For this review, take the finished solid that the model builds, in its own axes (mm). Give positions to 0.01 mm unless a question says otherwise; leave off trailing zeros. Write each loop counter-clockwise with the first axis right and the second up, starting at its lowest first coordinate (ties: lowest second). Pieces come first, ordered by that corner, then holes.
Q1. We need section C-C (z = 1.05). Write out the cut boundary in (x, y), then the cut area to 3 significant figures.
Q2. We need section A-A (y = 10). Write out the cut boundary in (x, z), then the cut area to 3 significant figures.
Q3. Insertion check: P1, Ø1.5, axis at x = -17, z = 1, coming from the -Y side; P2, Ø5, axis at x = -10, y = 10, coming from the +Z side. Each pin has a flat end and moves straight along its axis. Give the tip position at first contact, or say it passes through.
Q4. We need section B-B (x = -10). Write out the cut boundary in (y, z).
Q5. We need section D-D (y = 55). Write out the cut boundary in (x, z).
Q6. For line 1 (Y direction, x = -10, z = 0.6); line 2 (Y direction, x = -12.5, z = 0.25); line 3 (X direction, y = 13.5, z = 2.2), list the stretches that pass through material, from the lowest coordinate up.
Autodesk Inventor part; units mm, degrees
ref_plane "YZ Plane" through (0, 0, 0) normal (1, 0, 0) x (0, 1, 0)
ref_plane "XZ Plane" through (0, 0, 0) normal (0, 1, 0) x (-1, 0, 0)
ref_plane "XY Plane" through (0, 0, 0) normal (0, 0, 1) x (1, 0, 0)
sketch "Sketch1" plane through (0, 0, 0) normal (0, 0, 1) x (1, 0, 0)
  line L0 (-5, 65) -> (-15, 65)
  arc A0 (-15, 65) -> (-20, 60) centre (-15, 60) ccw
  line L1 (-20, 60) -> (-20, 5)
  arc A1 (-20, 5) -> (-15, 0) centre (-15, 5) ccw
  line L2 (-15, 0) -> (-5, 0)
  arc A2 (-5, 0) -> (0, 5) centre (-5, 5) ccw
  line L3 (0, 5) -> (0, 60)
  arc A3 (0, 60) -> (-5, 65) centre (-5, 60) ccw
  circle A4 centre (-10, 10) radius 4.3
  circle A5 centre (-10, 55) radius 4
  point P0 (0, 0)
  point P1 (0, 0)
  dimension "d0" = 8
  dimension "d1" = 8.6
extrude "Plate1" add sketch "Sketch1" along normal blind 2.5
equation "\"d2\" = Thickness"
equation "\"BendRadius\" = Thickness"
equation "\"BendReliefWidth\" = Thickness"
equation "\"BendReliefDepth\" = 0.5 * Thickness"
equation "\"MinimumRemnant\" = 2 * Thickness"
equation "\"TransitionRadius\" = BendRadius"
equation "\"JacobiRadiusSize\" = BendRadius"
equation "\"GapSize\" = Thickness"
properties part number "Servo horn"
Computed:
1. outline: (-20, 5) arc R5 ccw to (-15, 0) - (-5, 0) arc R5 ccw to (0, 5) - (0, 60) arc R5 ccw to (-5, 65) - (-15, 65) arc R5 ccw to (-20, 60) - close; hole circle Ø8.6 at (-10, 10); hole circle Ø8 at (-10, 55)
1. area: 1,170 mm2
2. outline: (-20, 0) - (-14.3, 0) - (-14.3, 2.5) - (-20, 2.5) - close; (-5.7, 0) - (0, 0) - (0, 2.5) - (-5.7, 2.5) - close
2. area: 28.5 mm2
3. P1: stops at y = 0.16
3. P2: passes through
4. outline: (0, 0) - (5.7, 0) - (5.7, 2.5) - (0, 2.5) - close; (14.3, 0) - (51, 0) - (51, 2.5) - (14.3, 2.5) - close; (59, 0) - (65, 0) - (65, 2.5) - (59, 2.5) - close
5. outline: (-20, 0) - (-14, 0) - (-14, 2.5) - (-20, 2.5) - close; (-6, 0) - (0, 0) - (0, 2.5) - (-6, 2.5) - close
6. line 1: y = 0 to 5.7, 14.3 to 51, 59 to 65
6. line 2: y = 0 to 6.5, 13.5 to 51.88, 58.12 to 65
6. line 3: x = -20 to -12.5, -7.5 to 0
